Drawing for the job (mm, zero at the part's lowest x, y, z). A direction names the side the tool comes from. Give positions to 0.01 mm unless a question says otherwise; leave off trailing zeros. Loops run counter-clockwise (first coordinate to the right, second up) from the corner with the lowest first, then second, coordinate; pieces in that order, holes last. Notation, with made-up numbers: (27, 85.5) -> (37, 85.5) arc R10 cw to (37, 101.5) -> close; hole circle Ø8 at (-20.5, 36.5). An arc over 180 degrees is marked (long way). Use CSV: the item, a comma, the result in double quotes. Start each with the question number.
(1) Drill centre lines: probe 1 along Z at (x, y) = (0.5, 2.7); probe 2 along X at (y, z) = (0.95, 4.4); probe 3 along Y at (x, z) = (8.75, 1.55). Where is each one in solid material? Low to high.
(2) Flat gauge pins, fed straight in: pin 1 (0.6 mm diameter, centred on x = 0.5, y = 3, fed in from +Z); pin 2 (0.6 mm diameter, centred on y = 3, z = 2.5, fed in from -X); pin 3 (1.5 mm diameter, centred on x = 7.5, z = 3.5, fed in from -Y). Where does each tip first touch, or does it go through?
(3) 3-axis set-ups, long thin cutter, end or side, ignore diameter. For the marked faces 4, 5 and 6: which of +Z, -Z, +X, -X, +Y, -Y reach the whole face in a straight line?
(4) Pull direction Y, two halves, no side cores. Call the marked faces 1, 2 and 3: pulls with the +Y half, pulls with the -Y half, needs draft (parallel to the pull), parting line crosses it, or undercut.
(5) Cut at B-B on x = 6.75. Write the cut outline in (y, z).
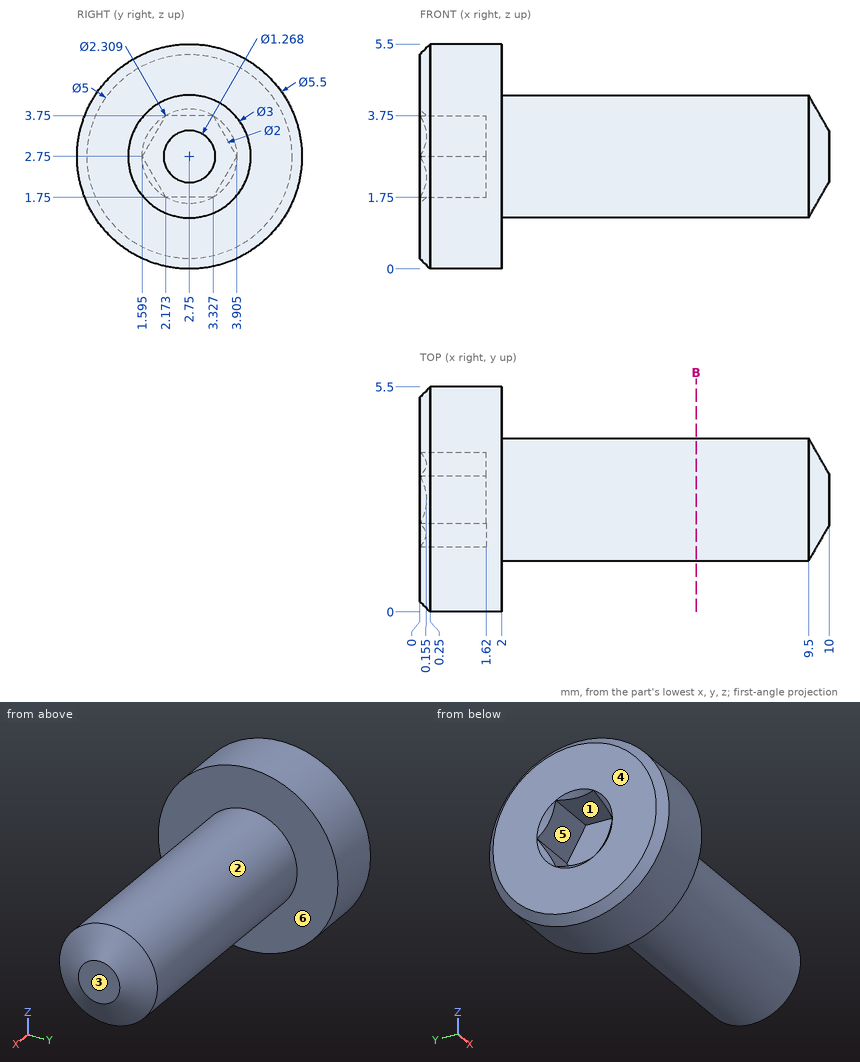
Check result:
1,probe 1,"0 to 1.75, 3.75 to 5.5"
1,probe 2,"0 to 2"
1,probe 3,"1.85 to 3.65"
2,pin 1,"z = 5.5"
2,pin 2,"x = 1.62"
2,pin 3,"y = 1.25"
3,face 4,"+Z, -Z, -X, +Y, -Y"
3,face 5,"-X"
3,face 6,"+X"
4,face 1,"undercut"
4,face 2,"parting line crosses it"
4,face 3,"needs draft"
5,outline,"circle Ø3 at (2.75, 2.75)"
